For this review, take the finished solid that the model builds, in its own axes (mm). A direction names the side the tool comes from. Coordinates: 2 decimals unless noted, no trailing zeros. Answer in a Markdown table with one row per item.
from build123d import *

# Parameters (mm, degrees)
BOSS_EXTRU_2_DEPTH      = 9
ESQUISSE3_R             = 9.644620121
ENL_V_MAT_EXTRU_1_DEPTH = 7
ESQUISSE5_R             = 7.8
ENL_V_MAT_EXTRU_2_DEPTH = 6
ESQUISSE6_W             = 99.948483018
ESQUISSE6_H             = 60
BOSS_EXTRU_3_DEPTH      = 5
ESQUISSE7_W             = 40
ESQUISSE7_H             = 39.978494119
BOSS_EXTRU_4_DEPTH      = 8
ENL_V_START             = -6.48388
ESQUISSE8_R             = 11
ENL_V_MAT_EXTRU_3_DEPTH = 6.48388
ESQUISSE9_R             = 8.165208678
ENL_V_MAT_EXTRU_4_DEPTH = 5
BOSS_EXTRU_5_DEPTH      = 99.948483018
BOSS_EXTRU_6_DEPTH      = 4
ENL_V_START_2           = -9
ENL_V_MAT_EXTRU_5_DEPTH = 9


with BuildPart() as part:
    # Esquisse2 → Boss.-Extru.2 (new body)
    with BuildSketch(Plane.ZY):
        with BuildLine():
            Line((142.883448923, 63.538611727), (142.883448923, 43.560117608))
            Line((142.883448923, 43.560117608), (142.883448923, 28.560117608))
            ThreePointArc((142.883448923, 28.560117608), (142.005344344, 24.462432419), (139.52524414, 21.084386454))
            ThreePointArc((139.52524414, 21.084386454), (136.436102048, 19.212462514), (132.883448923, 18.560117608))
            Line((132.883448923, 18.560117608), (192.883448923, 18.560117608))
            ThreePointArc((192.883448923, 18.560117608), (185.812381111, 21.489049797), (182.883448923, 28.560117608))
            Line((182.883448923, 28.560117608), (182.883448923, 43.560117608))
            Line((182.883448923, 43.560117608), (182.883448923, 63.538611727))
            Line((182.883448923, 63.538611727), (163.81068824, 63.538611727))
            Line((163.81068824, 63.538611727), (161.956209605, 63.538611727))
            Line((161.956209605, 63.538611727), (142.883448923, 63.538611727))
        make_face()
    extrude(amount=-BOSS_EXTRU_2_DEPTH)

    # Esquisse3 → Enlèv. mat.-Extru.1 (cut)
    with BuildSketch(Plane.ZY):
        with Locations((162.883448923, 43.560117608)):
            Circle(ESQUISSE3_R)
    extrude(amount=-ENL_V_MAT_EXTRU_1_DEPTH, mode=Mode.SUBTRACT)

    # Esquisse5 → Enlèv. mat.-Extru.2 (cut)
    with BuildSketch(Plane(origin=(9, 0, 0), x_dir=(0, 0, -1), z_dir=(1, 0, 0))):
        with Locations((-162.883448923, 43.560117608)):
            Circle(ESQUISSE5_R)
    extrude(amount=-ENL_V_MAT_EXTRU_2_DEPTH, mode=Mode.SUBTRACT)

    # Esquisse6 → Boss.-Extru.3 (add)
    with BuildSketch(Plane.XZ.offset(-18.560117608)):
        with Locations((49.974241509, 162.883448923)):
            Rectangle(ESQUISSE6_W, ESQUISSE6_H)
    extrude(amount=-BOSS_EXTRU_3_DEPTH)

    # Esquisse7 → Boss.-Extru.4 (add)
    with BuildSketch(Plane(origin=(69, 0, 0), x_dir=(0, 0, -1), z_dir=(1, 0, 0))):
        with Locations((-162.883448923, 43.549364668)):
            Rectangle(ESQUISSE7_W, ESQUISSE7_H)
    extrude(amount=-BOSS_EXTRU_4_DEPTH)

    # Esquisse8 → Enlèv. mat.-Extru.3 (cut)
    with BuildSketch(Plane(origin=(69, 0, 0), x_dir=(0, 0, -1), z_dir=(1, 0, 0)).offset(ENL_V_START)):
        with Locations((-162.883448923, 43.560117608)):
            Circle(ESQUISSE8_R)
    extrude(amount=ENL_V_MAT_EXTRU_3_DEPTH, mode=Mode.SUBTRACT)

    # Esquisse9 → Enlèv. mat.-Extru.4 (cut)
    with BuildSketch(Plane.ZY.offset(-61)):
        with Locations((162.883448923, 43.560117608)):
            Circle(ESQUISSE9_R)
    extrude(amount=-ENL_V_MAT_EXTRU_4_DEPTH, mode=Mode.SUBTRACT)

    # Esquisse10 → Boss.-Extru.5 (add)
    with BuildSketch(Plane(origin=(99.948483018, 0, 0), x_dir=(0, 0, -1), z_dir=(1, 0, 0))):
        with BuildLine():
            Line((-97.883448923, 69.817685904), (-100.410150097, 69.817685904))
            add(Edge.make_bspline(
                [(-100.410150097, 69.817685904), (-100.442033213, 68.80607378), (-100.50563029, 66.760024387), (-100.63239049, 62.850470513), (-100.810316501, 58.185123949), (-101.105084062, 52.996004141), (-101.670642078, 46.633188552), (-102.817961278, 39.776477829), (-104.76530294, 34.527578685), (-106.865826561, 31.248687809), (-108.756421045, 29.177953286), (-111.059219045, 27.42366281), (-113.90944146, 25.950331771), (-117.143373053, 24.872521409), (-119.940370542, 24.290171621), (-122.233093244, 23.949469798), (-124.260913893, 23.72661052), (-126.900847008, 23.559278589), (-129.29031887, 23.506975385), (-131.301500979, 23.518901656), (-132.360719769, 23.543642683), (-132.883448923, 23.560117608)],
                knots=[0, 0, 0, 0, 0.03125, 0.0625, 0.125, 0.1875, 0.25, 0.375, 0.5, 0.5625, 0.625, 0.6875, 0.75, 0.8125, 0.859709617, 0.875334617, 0.90625, 0.9375, 0.96875, 0.984375, 1, 1, 1, 1], degree=3))
            Line((-132.883448923, 23.560117608), (-192.883448923, 23.560117608))
            add(Edge.make_bspline(
                [(-192.883448923, 23.560117608), (-193.406178076, 23.543642683), (-194.465396866, 23.518901656), (-196.476578975, 23.506975385), (-198.866050837, 23.559278589), (-201.50594164, 23.726607838), (-203.533727382, 23.949460813), (-205.826459718, 24.290158055), (-208.623496676, 24.872512038), (-211.857456385, 25.950331771), (-214.7076788, 27.42366281), (-217.0104768, 29.177953286), (-218.901071284, 31.248687809), (-221.001594905, 34.527578685), (-222.948936567, 39.776477829), (-224.096255768, 46.633188552), (-224.661813783, 52.996004141), (-224.956581344, 58.185123949), (-225.134507355, 62.850470513), (-225.261267555, 66.760024387), (-225.324864632, 68.80607378), (-225.356747748, 69.817685904)],
                knots=[0, 0, 0, 0, 0.015625, 0.03125, 0.0625, 0.09375, 0.124663886, 0.140288886, 0.1875, 0.25, 0.3125, 0.375, 0.4375, 0.5, 0.625, 0.75, 0.8125, 0.875, 0.9375, 0.96875, 1, 1, 1, 1], degree=3))
            Line((-225.356747748, 69.817685904), (-227.883448923, 69.817685904))
            add(Edge.make_bspline(
                [(-227.883448923, 69.817685904), (-227.883448923, 36.967980152), (-228.338510952, 18.560117608), (-192.883448923, 18.560117608)],
                knots=[0, 0, 0, 0, 1, 1, 1, 1], degree=3))
            Line((-192.883448923, 18.560117608), (-132.883448923, 18.560117608))
            add(Edge.make_bspline(
                [(-97.883448923, 69.817685904), (-97.883448923, 36.967980152), (-97.428386893, 18.560117608), (-132.883448923, 18.560117608)],
                knots=[0, 0, 0, 0, 1, 1, 1, 1], degree=3))
        make_face()
    extrude(amount=-BOSS_EXTRU_5_DEPTH)

    # Esquisse11 → Boss.-Extru.6 (add)
    with BuildSketch(Plane.ZY):
        with BuildLine():
            Line((225.356747748, 69.817685904), (100.410150097, 69.817685904))
            add(Edge.make_bspline(
                [(100.410150097, 69.817685904), (100.442033213, 68.80607378), (100.50563029, 66.760024387), (100.63239049, 62.850470513), (100.810316501, 58.185123949), (101.105084062, 52.996004141), (101.670642078, 46.633188552), (102.817961278, 39.776477829), (104.76530294, 34.527578685), (106.865826561, 31.248687809), (108.756421045, 29.177953286), (111.059219045, 27.42366281), (113.90944146, 25.950331771), (117.143373053, 24.872521409), (119.940370542, 24.290171621), (122.233093244, 23.949469798), (124.260913893, 23.72661052), (126.900847008, 23.559278589), (129.29031887, 23.506975385), (131.301500979, 23.518901656), (132.360719769, 23.543642683), (132.883448923, 23.560117608)],
                knots=[0, 0, 0, 0, 0.03125, 0.0625, 0.125, 0.1875, 0.25, 0.375, 0.5, 0.5625, 0.625, 0.6875, 0.75, 0.8125, 0.859709617, 0.875334617, 0.90625, 0.9375, 0.96875, 0.984375, 1, 1, 1, 1], degree=3))
            Line((132.883448923, 23.560117608), (141.54370296, 23.560117608))
            ThreePointArc((141.54370296, 23.560117608), (142.542707185, 25.971927157), (142.883448923, 28.560117608))
            Line((142.883448923, 28.560117608), (142.883448923, 63.538611727))
            Line((142.883448923, 63.538611727), (182.883448923, 63.538611727))
            Line((182.883448923, 63.538611727), (182.883448923, 28.560117608))
            ThreePointArc((182.883448923, 28.560117608), (183.22419066, 25.971927157), (184.223194885, 23.560117608))
            Line((184.223194885, 23.560117608), (192.883448923, 23.560117608))
            add(Edge.make_bspline(
                [(192.883448923, 23.560117608), (193.406178076, 23.543642683), (194.465396866, 23.518901656), (196.476578975, 23.506975385), (198.866050837, 23.559278589), (201.50594164, 23.726607838), (203.533727382, 23.949460813), (205.826459718, 24.290158055), (208.623496676, 24.872512038), (211.857456385, 25.950331771), (214.7076788, 27.42366281), (217.0104768, 29.177953286), (218.901071284, 31.248687809), (221.001594905, 34.527578685), (222.948936567, 39.776477829), (224.096255768, 46.633188552), (224.661813783, 52.996004141), (224.956581344, 58.185123949), (225.134507355, 62.850470513), (225.261267555, 66.760024387), (225.324864632, 68.80607378), (225.356747748, 69.817685904)],
                knots=[0, 0, 0, 0, 0.015625, 0.03125, 0.0625, 0.09375, 0.124663886, 0.140288886, 0.1875, 0.25, 0.3125, 0.375, 0.4375, 0.5, 0.625, 0.75, 0.8125, 0.875, 0.9375, 0.96875, 1, 1, 1, 1], degree=3))
        make_face()
    extrude(amount=-BOSS_EXTRU_6_DEPTH)

    # Esquisse12 → Enlèv. mat.-Extru.5 (cut)
    with BuildSketch(Plane.ZY.offset(ENL_V_START_2)):
        with BuildLine():
            ThreePointArc((163.014719877, 32.973509037), (155.990303326, 35.524070266), (152.400224234, 42.078391173))
            ThreePointArc((152.400224234, 42.078391173), (145.080424512, 47.585238943), (139.573576742, 40.265439221))
            ThreePointArc((139.573576742, 40.265439221), (147.556262152, 25.691642787), (163.175335174, 20.020367203))
            ThreePointArc((163.175335174, 20.020367203), (169.571598443, 26.577245769), (163.014719877, 32.973509037))
        make_face()
        with BuildLine():
            ThreePointArc((171.408584799, 50.713555978), (174.012223438, 43.560117608), (171.408584799, 36.406679239))
            ThreePointArc((171.408584799, 36.406679239), (171.655098465, 33.589015134), (174.472762571, 33.8355288))
            ThreePointArc((174.472762571, 33.8355288), (178.012223438, 43.560117608), (174.472762571, 53.284706416))
            ThreePointArc((174.472762571, 53.284706416), (171.655098465, 53.531220083), (171.408584799, 50.713555978))
        make_face()
    extrude(amount=ENL_V_MAT_EXTRU_5_DEPTH, mode=Mode.SUBTRACT)


solid = part.part
Item 1: For L1, parallel to Z at x = 65, y = 39.5; L2, parallel to Y at x = 61, z = 187.5; L3, parallel to X at y = 38.5, z = 146.5, list the stretches that pass through material, from the lowest coordinate up.
Worked answers:
| item | result |
|---|---|
| L1 | 99.54 to 103.14, 142.88 to 152.66, 173.11 to 182.88, 222.63 to 226.23 |
| L2 | 18.56 to 23.56 |
| L3 | 61 to 69 |
Item 2: For faces 1 (the flat face through (4, 68, 162)), 2 (the flat face through (99.948, 23, 163)), 3 (the flat face through (61, 35, 163)), 4 (the cylindrical face through (3.451, 34.145, 160.793)), 5 (the cylindrical face through (65.71, 39.35, 152.72)), list the 3-axis set-ups (+Z, -Z, +X, -X, +Y, -Y) from which the entire face can be reached by the end or side of a thin tool; tool diameter is ignored.
Worked answers:
| item | result |
|---|---|
| face 1 | +X, +Y |
| face 2 | +Z, -Z, +X, +Y, -Y |
| face 3 | +Y |
| face 4 | -X |
| face 5 | +X |
Item 3: Take a section at A-A, the plane y = 45. Count the separate pieces of the cut face and the enclosed holes in it, and give its area (3 significant figures).
Worked answers:
| item | result |
|---|---|
| separate pieces | 6 |
| enclosed holes | 0 |
| area | 1,230 mm² |
Item 4: The part is to be moulded in two halves that separate along Z. For faces 6 (the flat face through (49, 18.56, 162)), 7 (the cylindrical face through (4.563, 35.455, 156.072)), say which applies: +Z half, -Z half, draft (parallel to the pull), parting line (faces both ways), or undercut.
Worked answers:
| item | result |
|---|---|
| face 6 | draft |
| face 7 | undercut |
Item 5: Insertion check: pin 1 (2 mm diameter, centred on y = 27, z = 161, fed in from -X); pin 2 (3 mm diameter, centred on y = 37.5, z = 189, fed in from +X); pin 3 (21 mm diameter, centred on y = 43.56, z = 162.88, fed in from +X). Each pin has a flat end and moves straight along its axis. Give the tip position at first contact, or say it passes through.
Worked answers:
| item | result |
|---|---|
| pin 1 | x = 61 |
| pin 2 | x = 4 |
| pin 3 | x = 62.52 |
